from build123d import *

# Parameters (mm, degrees)
BOSS_EXTRUDE2_DEPTH = 15
SKETCH7_R           = 3
CUT_EXTRUDE3_DEPTH  = 99.043475892
CHAMFER1_SIZE       = 2


with BuildPart() as part:
    # Sketch5 → Boss-Extrude2 (new, symmetric)
    with BuildSketch(Plane.XY):
        with BuildLine():
            Line((15.0591361, -15.818420273), (0, -23.706539182))
            Line((0, -23.706539182), (0, -63.706539182))
            Line((0, -63.706539182), (6, -63.706539182))
            Line((6, -63.706539182), (6, -38.706539182))
            ThreePointArc((6, -38.706539182), (8.928932188, -31.63547137), (16, -28.706539182))
            Line((16, -28.706539182), (44.293460818, -28.706539182))
            ThreePointArc((44.293460818, -28.706539182), (64.592049338, -20.29858852), (73, 0))
            ThreePointArc((73, 0), (71.8467278, 7.191695517), (68.502566573, 13.662175164))
            ThreePointArc((68.502566573, 13.662175164), (68.128388929, 12.868245276), (68, 12))
            Line((68, 12), (68, 0))
            ThreePointArc((68, 0), (55.687961475, -17.077678246), (35.594767305, -10.793019549))
            Line((35.594767305, -10.793019549), (7.997092947, 26.041058175))
            ThreePointArc((7.997092947, 26.041058175), (6.512400975, 28.87720155), (6, 32.037180147))
            Line((6, 32.037180147), (6, 63.706539182))
            Line((6, 63.706539182), (0, 63.706539182))
            Line((0, 63.706539182), (0, 23.706539182))
            Line((0, 23.706539182), (17.168258803, -9.069227623))
            ThreePointArc((17.168258803, -9.069227623), (17.511501017, -12.880637562), (15.0591361, -15.818420273))
        make_face()
        with BuildLine():
            ThreePointArc((68, 12), (68.128388929, 12.868245276), (68.502566573, 13.662175164))
            ThreePointArc((68.502566573, 13.662175164), (62.293432752, 19.438917438), (54.41285467, 22.572698413))
            add(Edge.make_bspline(
                [(54.41285467, 22.572698413), (48.698801755, 23.689768452), (29.182846067, 17.084288793), (12.266368885, 20.342938845), (7.997092947, 26.041058175)],
                knots=[0, 0, 0, 0, 0.577740896, 1, 1, 1, 1], degree=3))
            Line((7.997092947, 26.041058175), (35.594767305, -10.793019549))
            ThreePointArc((35.594767305, -10.793019549), (44.312038525, 17.077678246), (68, 0))
            Line((68, 0), (68, 12))
        make_face()
    extrude(amount=BOSS_EXTRUDE2_DEPTH, both=True)

    # Sketch7 → Cut-Extrude3 (cut, through all)
    with BuildSketch(Plane(origin=(0, 0, 0), x_dir=(0, 0, -1), z_dir=(1, 0, 0))):
        with Locations(Location((0, -50, 0), (0, 0, 270))):
            Circle(SKETCH7_R)
        with Locations(Location((0, 50, 0), (0, 0, 90))):
            Circle(SKETCH7_R)
    extrude(amount=CUT_EXTRUDE3_DEPTH, mode=Mode.SUBTRACT)

    # Chamfer1
    chamfer1_edges = [part.edges().sort_by_distance(p)[0] for p in [
        (6, -63.706539182, 0),
        (6, 63.706539182, 0),
        (6, -47, 0),
        (6, 47, 0),
    ]]
    chamfer(chamfer1_edges, length=CHAMFER1_SIZE)


solid = part.part
Here's how the part is built. I have some questions about the finished solid (model axes, mm). A direction names the side the tool comes from. Round coordinates to 2 decimals unless told otherwise and drop trailing zeros. Loops run counter-clockwise (first coordinate to the right, second up) from the corner with the lowest first, then second, coordinate; pieces in that order, holes last. Notation, with made-up numbers: (77, 80.25) -> (121, 80.25) arc R27 cw to (121, 102.25) -> close; hole circle Ø11 at (42.5, 68.25). An arc over 180 degrees is marked (long way). Write each question's results on one line, items separated by ' | '.
(1) If we section it at D-D, the plane y = 37: List the corners of the cut face in (x, z) for me.
Worked answers:
outline: (0, -15) -> (6, -15) -> (6, 15) -> (0, 15) -> close
(2) If we section it at C-C, the plane z = -1.5: Give the number of separate pieces and of enclosed holes in the cut face, then the cut area to 3 significant figures.
Worked answers:
separate pieces: 3 | enclosed holes: 1 | area: 2,330 mm2
(3) For P1, Ø1.5, axis at y = -45.5, z = 0, coming from the +X side; P2, Ø12, axis at y = 6.5, z = 2, coming from the +X side; P3, Ø6, axis at y = -19, z = 4, coming from the -X side, each with a flat end and sliding along its axis, tell me the tip position at first contact or that it passes through.
Worked answers:
P1: x = 6 | P2: x = 72.99 | P3: x = 3.26
(4) If I drill on L1, parallel to Z at x = 1.8, y = -50; L2, parallel to Y at x = 49.5, z = 12; L3, parallel to Y at x = 11.5, z = -13, over which ranges is the centre line in solid material (lowest first)?
Worked answers:
L1: -15 to -3, 3 to 15 | L2: -28.23 to -17.99, 17.99 to 22.65 | L3: -29.78 to -17.68, 1.75 to 22.67
(5) We'd pull the mould along Z, two halves only. Please class faces 5 (the face through (23, -4, 15)), 6 (the face through (6.53, 28.83, 0.21)), 7 (the face through (2, -47, 0)), 8 (the face through (2, 47, 0)): released by +Z, released by -Z, zero draft, split by the parting line, or undercut.
Worked answers:
face 5: released by +Z | face 6: zero draft | face 7: undercut | face 8: undercut
(6) For faces 1 (the face through (2, 63.707, 0)), 2 (the face through (30, -28.707, 0)), 3 (the face through (8.464, 7.548, 0.21)), 4 (the face through (6, 43, 0)), which set-ups out of +Z, -Z, +X, -X, +Y, -Y let a thin tool reach every point of the face, with its end or its side?
Worked answers:
face 1: +Z, -Z, +X, -X, +Y | face 2: +Z, -Z, +X, -Y | face 3: +Z, -Z, -X | face 4: +Z, -Z, +X, +Y
(7) If we section it at B-B, the plane y = -14.5: List the corners of the cut face in (x, z) for me, then the cut area to 3 significant figures.
Worked answers:
outline: (16.65, -15) -> (39.33, -15) -> (39.33, 15) -> (16.65, 15) -> close; (60.67, -15) -> (69.07, -15) -> (69.07, 15) -> (60.67, 15) -> close | area: 933 mm2
(8) If we section it at A-A, the plane y = -50: List the corners of the cut face in (x, z) for me.
Worked answers:
outline: (0, -15) -> (6, -15) -> (6, -5) -> (4, -3) -> (0, -3) -> close; (0, 3) -> (4, 3) -> (6, 5) -> (6, 15) -> (0, 15) -> close
